Build history of the part. All positions in model axes, mm. Face numbers are marked on the shaded views. A direction names the side the tool comes from. Round coordinates to 2 decimals unless told otherwise and drop trailing zeros. Write each loop counter-clockwise with the first axis right and the second up, starting at its lowest first coordinate (ties: lowest second). Pieces come first, ordered by that corner, then holes. Notation, with made-up numbers: (83.25, 67.25) -> (114.25, 67.25) arc R26 cw to (114.25, 97.25) -> close; hole circle Ø11 at (42.25, -18.75). An arc over 180 degrees is marked (long way). Answer in a Markdown table with one row per item.
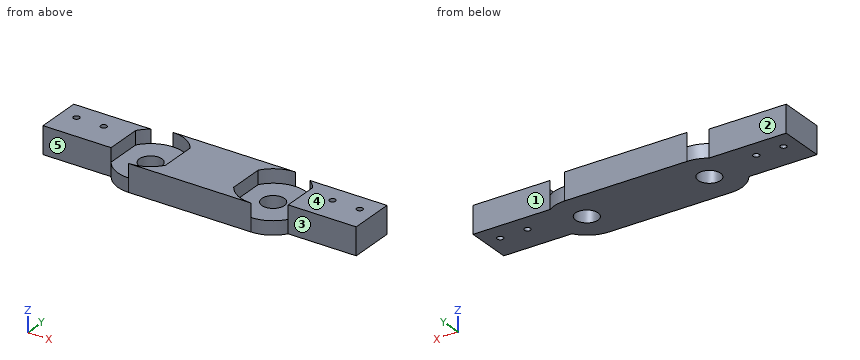
```python
from build123d import *

# Parameters (mm, degrees)
SKETCH_1_W                  = 130
SKETCH_1_H                  = 48
SKETCH_1_R                  = 8.25
EXTRUDE_1_DEPTH             = 10
CUT_EXTRUDE_1_DEPTH         = 10
EXTRUDE_START               = 10
EXTRUDE_2_DEPTH             = 10
SKETCH_6_W                  = 10
SKETCH_6_H                  = 26.532998322
EXTRUDE_3_DEPTH             = 50
SKETCH_7_W                  = 50
SKETCH_7_H                  = 26.532998322
EXTRUDE_4_DEPTH             = 10
HOLE_WIZARD_M4_1_AT_2_COUNT = 2
HOLE_WIZARD_M4_1_AT_2_PITCH = 20
EXTRUDE_6_DEPTH             = 20


with BuildPart() as part:
    # 스케치1 → 보스-돌출1 (new body)
    with BuildSketch(Plane.XY):
        with Locations((45, 0)):
            Rectangle(SKETCH_1_W, SKETCH_1_H)
        Circle(SKETCH_1_R, mode=Mode.SUBTRACT)
        with Locations((90, 0)):
            Circle(SKETCH_1_R, mode=Mode.SUBTRACT)
    extrude(amount=EXTRUDE_1_DEPTH)

    # 스케치4 → 컷-돌출1 (cut)
    with BuildSketch(Plane.XY.offset(10)):
        with BuildLine():
            Line((-20, 24), (-20, 13.266499161))
            ThreePointArc((-20, 13.266499161), (-11.349097324, 21.147056295), (0, 24))
            Line((0, 24), (-20, 24))
        make_face()
        with BuildLine():
            ThreePointArc((0, -24), (-11.349097324, -21.147056295), (-20, -13.266499161))
            Line((-20, -13.266499161), (-20, -24))
            Line((-20, -24), (0, -24))
        make_face()
        with BuildLine():
            ThreePointArc((110, -13.266499161), (101.349097324, -21.147056295), (90, -24))
            Line((90, -24), (110, -24))
            Line((110, -24), (110, -13.266499161))
        make_face()
        with BuildLine():
            Line((110, 24), (90, 24))
            ThreePointArc((90, 24), (101.349097324, 21.147056295), (110, 13.266499161))
            Line((110, 13.266499161), (110, 24))
        make_face()
    extrude(amount=-CUT_EXTRUDE_1_DEPTH, mode=Mode.SUBTRACT)

    # 스케치5 → 보스-돌출2 (add)
    with BuildSketch(Plane.XY.offset(10).offset(EXTRUDE_START)):
        with BuildLine():
            Line((20, -13.266499161), (20, 13.266499161))
            ThreePointArc((20, 13.266499161), (11.349097324, 21.147056295), (0, 24))
            Line((0, 24), (90, 24))
            ThreePointArc((90, 24), (78.650902676, 21.147056295), (70, 13.266499161))
            Line((70, 13.266499161), (70, -13.266499161))
            ThreePointArc((70, -13.266499161), (78.650902676, -21.147056295), (90, -24))
            Line((90, -24), (0, -24))
            ThreePointArc((0, -24), (11.349097324, -21.147056295), (20, -13.266499161))
        make_face()
    extrude(amount=-EXTRUDE_2_DEPTH)

    # 스케치6 → 보스-돌출3 (add)
    with BuildSketch(Plane(origin=(110, 0, 0), x_dir=(0, 0, -1), z_dir=(1, 0, 0))):
        with Locations((-5, 0)):
            Rectangle(SKETCH_6_W, SKETCH_6_H)
    extrude_3 = extrude(amount=EXTRUDE_3_DEPTH)

    # 스케치7 → 보스-돌출4 (add)
    with BuildSketch(Plane.XY.offset(10)):
        with Locations((135, 0)):
            Rectangle(SKETCH_7_W, SKETCH_7_H)
    extrude_4 = extrude(amount=EXTRUDE_4_DEPTH)

    # 대칭 복사2: 보스-돌출3, 보스-돌출4 across plane
    add(extrude_3.mirror(Plane.ZY.offset(-45)))
    add(extrude_4.mirror(Plane.ZY.offset(-45)))

    # 스케치11 → M4 남비 머리 나사용 카운터보어1 (revolve, cut)
    with BuildSketch(Plane(origin=(-59, 6.733500839, 30), x_dir=(0, -1, 0), z_dir=(1, 0, 0))):
        Polygon((0, 0), (0, 31.351936393), (2.25, 30), (2.25, 3.1), (4.5, 3.1), (4.5, 0), align=None)
    hole_wizard_m4_1 = revolve(axis=Axis((-59, 6.733500839, 36.35), (0, 0, -1)), mode=Mode.SUBTRACT)

    # M4 남비 머리 나사용 카운터보어1 at 2: M4 남비 머리 나사용 카운터보어1 ×2
    with Locations(*[(i * HOLE_WIZARD_M4_1_AT_2_PITCH, 0, 0) for i in range(1, HOLE_WIZARD_M4_1_AT_2_COUNT)]):
        add(hole_wizard_m4_1, mode=Mode.SUBTRACT)

    # 스케치14 → 보스-돌출6 (add, through all)
    with BuildSketch(Plane.XY.offset(20)):
        with BuildLine():
            ThreePointArc((-20, 13.266499161), (-16.991935867, 16.949162679), (-13.316865669, 19.966499161))
            Line((-13.316865669, 19.966499161), (-70, 19.966499161))
            Line((-70, 19.966499161), (-70, 13.266499161))
            Line((-70, 13.266499161), (-20, 13.266499161))
        make_face()
    extrude_6 = extrude(amount=-EXTRUDE_6_DEPTH)

    # 대칭 복사3: M4 남비 머리 나사용 카운터보어1, 보스-돌출6 across plane
    add(hole_wizard_m4_1.mirror(Plane.ZY.offset(-45)), mode=Mode.SUBTRACT)
    add(extrude_6.mirror(Plane.ZY.offset(-45)))

    # 대칭 복사3 copy 1 sketch → 대칭 복사3 copy 1 (revolve, cut)
    with BuildSketch(Plane(origin=(129, 6.733500839, 30), x_dir=(0, -1, 0), z_dir=(-1, 0, 0))):
        Polygon((0, 0), (0, -31.351936393), (2.25, -30), (2.25, -3.1), (4.5, -3.1), (4.5, 0), align=None)
    revolve(axis=Axis((129, 6.733500839, 36.35), (0, 0, 1)), mode=Mode.SUBTRACT)


solid = part.part
```
Q1. Which spindle directions (+Z, -Z, +X, -X, +Y, -Y) get a long thin tool onto all of the face, cutting with end or side? Do the marked faces 1, 2, 3, 4 and 5. Say none if no direction does.
A:
| item | result |
|---|---|
| face 1 | +Z, -Z, +X, +Y |
| face 2 | +Z, -Z, -X, +Y |
| face 3 | +Z, -Z, +X, -Y |
| face 4 | +Z, +X, -X, +Y, -Y |
| face 5 | +Z, -Z, -X, -Y |
Q2. Saw through at B-B on x = -59. Write the cut outline in (y, z), plus the area to 3 significant figures.
A:
| item | result |
|---|---|
| outline | (-13.27, 0) -> (4.48, 0) -> (4.48, 20) -> (-13.27, 20) -> close; (8.98, 0) -> (19.97, 0) -> (19.97, 20) -> (8.98, 20) -> close |
| area | 575 mm² |
Q3. Saw through at D-D on x = 5. Write the cut outline in (y, z).
A:
| item | result |
|---|---|
| outline | (-24, 0) -> (-6.56, 0) -> (-6.56, 10) -> (-23.47, 10) -> (-23.47, 20) -> (-24, 20) -> close; (6.56, 0) -> (24, 0) -> (24, 20) -> (23.47, 20) -> (23.47, 10) -> (6.56, 10) -> close |
Q4. Saw through at C-C on y = 0. Write the cut outline in (x, z), plus the area to 3 significant figures.
A:
| item | result |
|---|---|
| outline | (-70, 0) -> (-8.25, 0) -> (-8.25, 10) -> (-20, 10) -> (-20, 20) -> (-70, 20) -> close; (8.25, 0) -> (81.75, 0) -> (81.75, 10) -> (70, 10) -> (70, 20) -> (20, 20) -> (20, 10) -> (8.25, 10) -> close; (98.25, 0) -> (160, 0) -> (160, 20) -> (110, 20) -> (110, 10) -> (98.25, 10) -> close |
| area | 3,470 mm² |
Q5. Drop a flat-ended pin along its axis: P1, Ø20, axis at x = 87, y = -3, coming from the +Z side. Give the stop position or say it passes through.
A:
| item | result |
|---|---|
| P1 | z = 10 |
Q6. Wall check: line 1 (X direction, y = -9, z = 17.5); line 2 (Y direction, x = 129, z = 15.75); line 3 (X direction, y = -2, z = 3.25). Give the ranges that are in metal, low to high. Write a range as [from, to].
A:
| item | result |
|---|---|
| line 1 | [-70, -20], [20, 70], [110, 160] |
| line 2 | [-13.27, 4.48], [8.98, 19.97] |
| line 3 | [-70, -8], [8, 82], [98, 160] |
Q7. Saw through at A-A on z = 13. Write the cut outline in (x, y), plus the area to 3 significant figures.
A:
| item | result |
|---|---|
| outline | (-70, -13.27) -> (-20, -13.27) -> (-20, 13.27) arc R24 cw to (-13.32, 19.97) -> (-70, 19.97) -> close; (0, -24) -> (90, -24) arc R24 cw to (70, -13.27) -> (70, 13.27) arc R24 cw to (90, 24) -> (0, 24) arc R24 cw to (20, 13.27) -> (20, -13.27) arc R24 cw to start; (103.32, 19.97) arc R24 cw to (110, 13.27) -> (110, -13.27) -> (160, -13.27) -> (160, 19.97) -> close; hole circle Ø4.5 at (-59, 6.73); hole circle Ø4.5 at (-39, 6.73); hole circle Ø4.5 at (129, 6.73); hole circle Ø4.5 at (149, 6.73) |
| area | 5,950 mm² |
